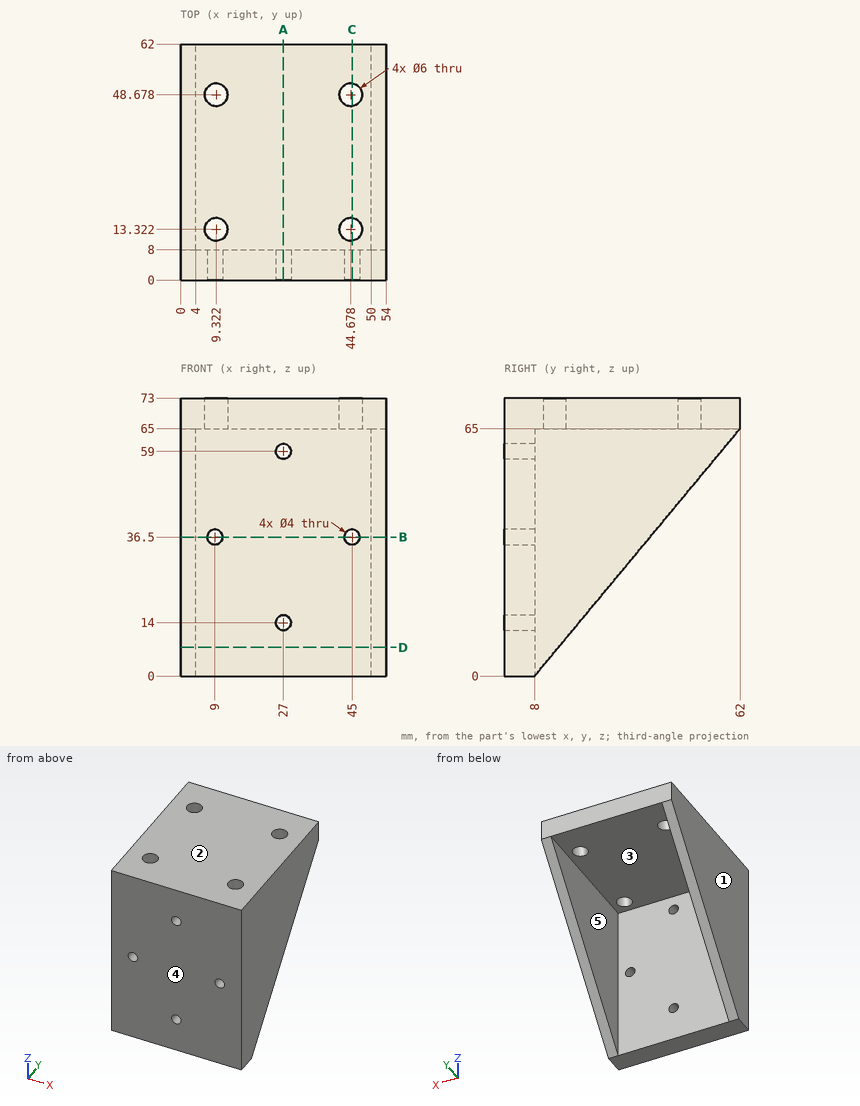
Check sheet for the drawn part. Datum: minimum x, y, z corner. Units: mm. A direction names the side the tool comes from. Round coordinates to 2 decimals unless told otherwise and drop trailing zeros. Loops run counter-clockwise (first coordinate to the right, second up) from the corner with the lowest first, then second, coordinate; pieces in that order, holes last. Notation, with made-up numbers: (87, 8) -> (114, 8) arc R12 ccw to (114, 22) -> close; hole circle Ø6 at (-32, 3.5). An arc over 180 degrees is marked (long way). Put each result on its own line as item: value. Start each with the question number.
1. Access from +Z, -Z, +X, -X, +Y, -Y to the whole of each face (thin tool, end or side, straight path). Record for the marked faces 4 and 5.
2. Section check D-D (z = 7.5). Enter the section's corners in (x, y), plus the area to 3 significant figures.
3. Scan lines: probe 1 along Z at (x, y) = (27, 6.5); probe 2 along X at (y, z) = (22.5, 31); probe 3 along Z at (x, y) = (45, 5). Record each from-to range of solid material in increasing order.
4. Gauge pin test, flat end, axial feed: pin 1 (1.5 mm diameter, centred on x = 21.5, z = 44.5, fed in from +Y). Record the tip position at first contact, or that the pin passes through.
5. Section check A-A (x = 27). Enter the section's corners in (y, z), plus the area to 3 significant figures.
6. Section check B-B (z = 36.5). Enter the section's corners in (x, y).
7. Draft check along X on the marked faces 1, 2 and 3. Enter one of: +X half, -X half, draft (parallel to the pull), parting line (faces both ways), or undercut.
8. Section check C-C (x = 45). Enter the section's corners in (y, z) (1 decimal).
Findings:
1. face 4: +Z, -Z, +X, -X, -Y
1. face 5: -Z, +Y
2. outline: (0, 0) -> (54, 0) -> (54, 14.23) -> (50, 14.23) -> (50, 8) -> (4, 8) -> (4, 14.23) -> (0, 14.23) -> close
2. area: 482 mm^2
3. probe 1: z = 0 to 12, 16 to 57, 61 to 73
3. probe 2: x = 0 to 4, 50 to 54
3. probe 3: z = 0 to 34.5, 38.5 to 73
4. pin 1: stops at y = 8
5. outline: (0, 0) -> (8, 0) -> (8, 12) -> (0, 12) -> close; (0, 16) -> (8, 16) -> (8, 57) -> (0, 57) -> close; (0, 61) -> (8, 61) -> (8, 65) -> (62, 65) -> (62, 73) -> (0, 73) -> close
5. area: 952 mm^2
6. outline: (0, 0) -> (7, 0) -> (7, 8) -> (4, 8) -> (4, 38.32) -> (0, 38.32) -> close; (11, 0) -> (43, 0) -> (43, 8) -> (11, 8) -> close; (47, 0) -> (54, 0) -> (54, 38.32) -> (50, 38.32) -> (50, 8) -> (47, 8) -> close
7. face 1: -X half
7. face 2: draft
7. face 3: undercut
8. outline: (0, 0) -> (8, 0) -> (8, 34.5) -> (0, 34.5) -> close; (0, 38.5) -> (8, 38.5) -> (8, 65) -> (10.3, 65) -> (10.3, 73) -> (0, 73) -> close; (16.3, 65) -> (45.7, 65) -> (45.7, 73) -> (16.3, 73) -> close; (51.7, 65) -> (62, 65) -> (62, 73) -> (51.7, 73) -> close
